```python
from build123d import *

# Parameters (mm, degrees)
F_1_8_0_125_DIAMETER_HOLE1_D     = 3.175
F_1_8_0_125_DIAMETER_HOLE1_DEPTH = 0.011333767
F_1_8_0_125_DIAMETER_HOLE1_TIP   = 0.953866233


with BuildPart() as part:
    # Sketch1 → Revolve1 (revolve)
    with BuildSketch(Plane.XY, mode=Mode.PRIVATE) as revolve1_sk:
        Polygon((0, 4.7625), (3.175, 4.7625), (3.175, 0.79375), (6.35, 0.79375), (6.35, -0.79375), (3.175, -0.79375), (3.175, -4.7625), (0, -4.7625), align=None)
    revolve(revolve1_sk.sketch.rotate(Axis((0, 4.7625, 0), (0, -1, 0)), 90), axis=Axis((0, 4.7625, 0), (0, -1, 0)))

    # 1/8 (0.125) Diameter Hole1
    with Locations(Plane(origin=(0, 4.7625, 0), x_dir=(1, 0, 0), z_dir=(0, 1, 0))):
        with Locations((0, 0)):
            Hole(F_1_8_0_125_DIAMETER_HOLE1_D / 2, depth=F_1_8_0_125_DIAMETER_HOLE1_DEPTH)
            with Locations((0, 0, -(F_1_8_0_125_DIAMETER_HOLE1_DEPTH + F_1_8_0_125_DIAMETER_HOLE1_TIP / 2))):  # 118° drill point
                Cone(0, F_1_8_0_125_DIAMETER_HOLE1_D / 2, F_1_8_0_125_DIAMETER_HOLE1_TIP, mode=Mode.SUBTRACT)


solid = part.part
```
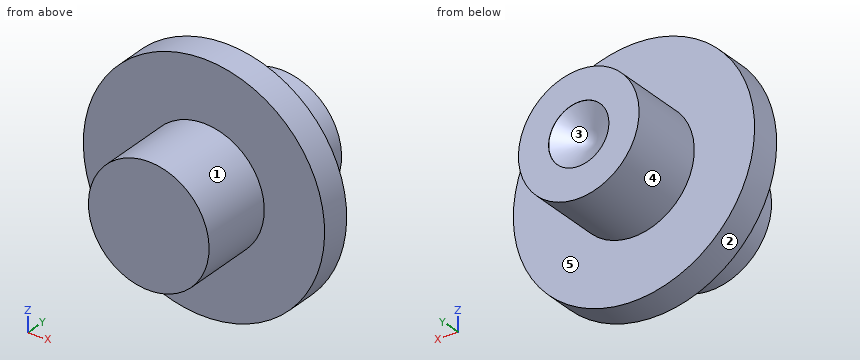
The model under review builds one solid part; all positions refer to its coordinate system, in mm. Face numbers are marked on the shaded views. A direction names the side the tool comes from. Round coordinates to 2 decimals unless told otherwise and drop trailing zeros. Loops run counter-clockwise (first coordinate to the right, second up) from the corner with the lowest first, then second, coordinate; pieces in that order, holes last. Notation, with made-up numbers: M -14,46.25 L 12,46.25 A21 cw 12,59.25 Z; hole C 7,15 d2. An arc over 180 degrees is marked long. Put each result on its own line as item: value.
Q1. Machinability: for the marked faces 1 and 2, which of the approach directions +Z, -Z, +X, -X, +Y, -Y give a long, thin tool a straight path to every point of the face, cutting with its end or side? Answer none if there is none.
Result set:
face 1: -Y
face 2: +Y, -Y
Q2. Consider section D-D, the plane z = -4. Give the boundary of the cut face in (x, y), then the cut area to 3 significant figures.
Result set:
outline: M -4.93,-0.79 L 4.93,-0.79 L 4.93,0.79 L -4.93,0.79 Z
area: 15.7 mm²
Q3. Consider section B-B, the plane x = -2.75. Give the boundary of the cut face in (y, z).
Result set:
outline: M -4.76,-1.59 L -0.79,-1.59 L -0.79,-5.72 L 0.79,-5.72 L 0.79,-1.59 L 4.76,-1.59 L 4.76,1.59 L 0.79,1.59 L 0.79,5.72 L -0.79,5.72 L -0.79,1.59 L -4.76,1.59 Z
Q4. Consider section A-A, the plane z = -2.5. Give the boundary of the cut face in (x, y), then the cut area to 3 significant figures.
Result set:
outline: M -5.84,-0.79 L -1.96,-0.79 L -1.96,-4.76 L 1.96,-4.76 L 1.96,-0.79 L 5.84,-0.79 L 5.84,0.79 L 1.96,0.79 L 1.96,4.76 L -1.96,4.76 L -1.96,0.79 L -5.84,0.79 Z
area: 49.6 mm²
Q5. To check wall thickness, follow L1, parallel to Y at x = -5.5, z = -0.75; L2, parallel to X at y = 4.25, z = -0.5; L3, parallel to X at y = 0.5, z = -5.5. State the ranges of each line that lie inside material, in increasing order.
Result set:
L1: y = -0.79 to 0.79
L2: x = -3.14 to -0.56, 0.56 to 3.14
L3: x = -3.17 to 3.17
Q6. For pin 1 (1 mm diameter, centred on x = 1, z = 4.5, fed in from -Y); pin 2 (3 mm diameter, centred on y = 3, z = 1.5, fed in from +X) (3 decimals); pin 3 (4 mm diameter, centred on y = 0, z = -5, fed in from +X), all flat-tipped, find the tip position at first contact; note any pin that passes through.
Result set:
pin 1: stops at y = -0.79
pin 2: stops at x = 3.175
pin 3: stops at x = 5.6
Q7. Consider section C-C, the plane y = -4. Give the boundary of the cut face in (x, z) (3 decimals).
Result set:
outline: C 0,0 d6.35
Q8. Mouldability with a two-part tool opening along Z and no side actions: class the marked faces 3, 4 and 5 as released by +Z, released by -Z, zero draft, split by the parting line, or undercut.
Result set:
face 3: undercut
face 4: split by the parting line
face 5: zero draft
